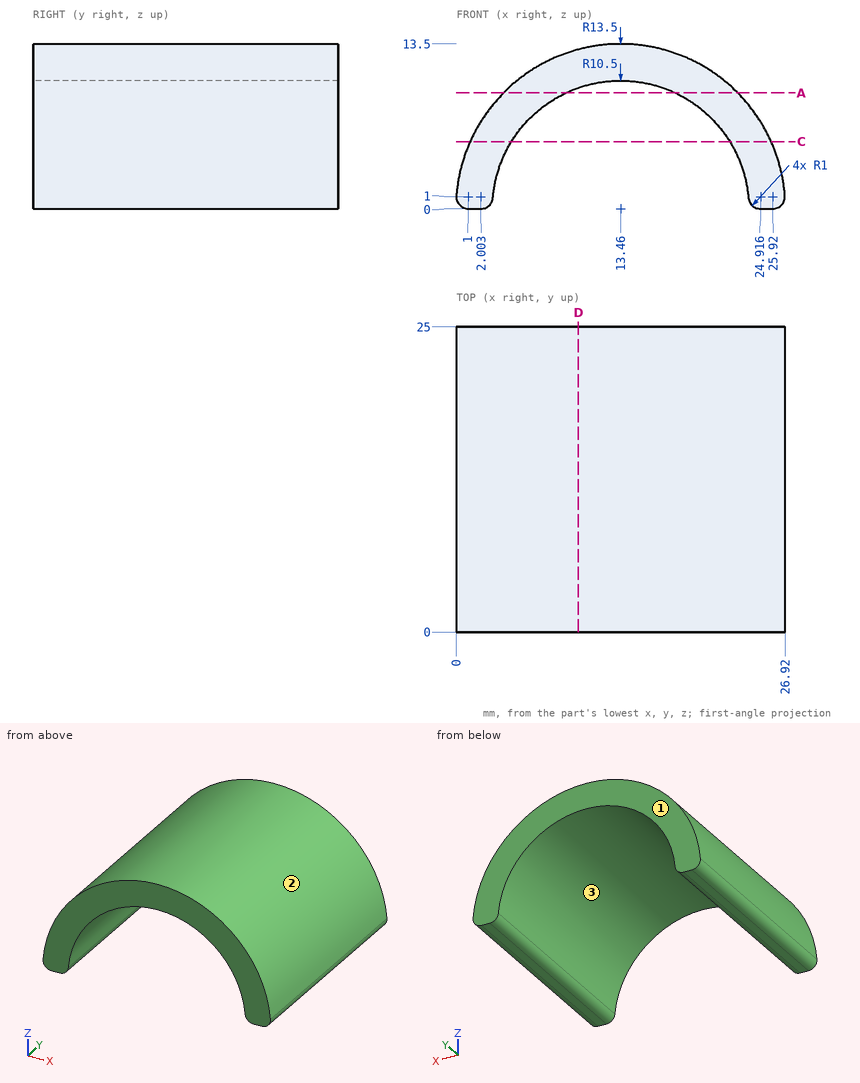
Check sheet for the drawn part. Datum: minimum x, y, z corner. Units: mm. Coordinates: 2 decimals unless noted, no trailing zeros. Order: outer loops, then holes, each group sorted by start corner. A loop starts at its lowest first (then second) coordinate and runs counter-clockwise, first axis right, second up. Notation, with made-up numbers: (-4, 53) -> (6, 53) arc R11 ccw to (6, 64) -> close; hole circle Ø7 at (82.5, 32). An arc over 180 degrees is marked (long way). Use a Markdown table: item, result. Add a question column.
1. Cross-section at A-A (z = 9.5). Enter the section's corners in (x, y).
2. Go/stop test with flat-tipped pins: pin 1 Ø5 at (y, z) = (4, 8.5) entering from +X; pin 2 Ø5 at (x, y) = (5, 5.5) entering from +Z; pin 3 Ø2 at (y, z) = (13.5, 3.5) entering from -X; pin 4 Ø5 at (x, z) = (20, 2) entering from -Y. Record where each tip stops, or that it passes through.
3. Cross-section at D-D (x = 10). Enter the section's corners in (y, z).
4. Cross-section at C-C (z = 5.5). Enter the section's corners in (x, y) (1 decimal), and give its area (3 significant figures).
5. Material ranges on L1, parallel to X at y = 6.5, z = 1.5; L2, parallel to X at y = 9.25, z = 3.25 (1 decimal); L3, parallel to Z at x = 13.75, y = 15.25 (1 decimal), recorded low to high.
6. Mould release check, pull along X, two halves, no side actions. Record for the marked faces 1, 2 and 3: pulls with the +X half, pulls with the -X half, needs draft (parallel to the pull), parting line crosses it, or undercut.
Filled sheet:
| question | item | result |
|---|---|---|
| 1 | outline | (3.87, 0) -> (8.99, 0) -> (8.99, 25) -> (3.87, 25) -> close; (17.93, 0) -> (23.05, 0) -> (23.05, 25) -> (17.93, 25) -> close |
| 2 | pin 1 | x = 25.55 |
| 2 | pin 2 | z = 12.11 |
| 2 | pin 3 | x = 0.19 |
| 2 | pin 4 | through |
| 3 | outline | (0, 9.91) -> (25, 9.91) -> (25, 13.05) -> (0, 13.05) -> close |
| 4 | outline | (1.1, 0) -> (4.5, 0) -> (4.5, 25) -> (1.1, 25) -> close; (22.4, 0) -> (25.8, 0) -> (25.8, 25) -> (22.4, 25) -> close |
| 4 | area | 169 mm2 |
| 5 | L1 | 0.04 to 3.07, 23.85 to 26.88 |
| 5 | L2 | 0.4 to 3.5, 23.4 to 26.6 |
| 5 | L3 | 10.5 to 13.5 |
| 6 | face 1 | needs draft |
| 6 | face 2 | parting line crosses it |
| 6 | face 3 | undercut |
